Here's how the part is built. I have some questions about the finished solid (model axes, mm). A direction names the side the tool comes from. Round coordinates to 2 decimals unless told otherwise and drop trailing zeros. Write item = value, one per line. Start each with the question number.
Item 1: For faces 4 (the face through (33, -1.27, -17)), 5 (the face through (0.018, 27.397, 10.874)), 6 (the face through (-27.397, 0.018, 10.874)), 7 (the face through (-33, 1.27, -17)), which set-ups out of +Z, -Z, +X, -X, +Y, -Y let a thin tool reach every point of the face, with its end or its side?
Item 2: We'd pull the mould along Z, two halves only. Please class faces 1 (the face through (-6.21, -1.96, -88.74)), 2 (the face through (1.27, 33, -17)), 3 (the face through (-1.9, -8.7, -2.4)): pulls with the +Z half, pulls with the -Z half, needs draft (parallel to the pull), parting line crosses it, or undercut.
Item 3: I'm going to push flat-ended pins straight in: P1, Ø0.6, axis at x = 16.5, z = -102, coming from the -Y side; P2, Ø12.5, axis at x = 1.5, y = 4.5, coming from the +Z side; P3, Ø3, axis at x = 5.5, y = -32.5, coming from the +Z side. Where does each tip first touch, or does it pass through?
Item 4: Please list where these lines run through material, in increasing order: L1, parallel to X at y = 43.5, z = -3.5; L2, parallel to Z at x = 26, y = -9.
```python
from build123d import *

# Parameters (mm, degrees)
SKETCH2_R           = 8.763
CUT_EXTRUDE1_DEPTH  = 69.85
BOSS_EXTRUDE1_DEPTH = 1.27
CIRPATTERN1_COUNT   = 4
CHAMFER1_SIZE       = 2.54
SKETCH10_W          = 76.2
SKETCH10_H          = 76.2
BOSS_EXTRUDE4_DEPTH = 0.508


with BuildPart() as part:
    # Sketch1 → Revolve1 (revolve)
    with BuildSketch(Plane(origin=(0, 0, 0), x_dir=(1, 0, 0), z_dir=(0, 1, 0))):
        Polygon((0, 101.6), (-6.096, 101.6), (-6.096, 89.154), (-12.7, 82.55), (-12.7, 0), (0, 0), align=None)
    revolve(axis=Axis((0, 0, -101.6), (0, 0, 1)))

    # Sketch2 → Cut-Extrude1 (cut)
    with BuildSketch(Plane.XY):
        Circle(SKETCH2_R)
    extrude(amount=-CUT_EXTRUDE1_DEPTH, mode=Mode.SUBTRACT)

    # Sketch3 → Boss-Extrude1 (add, symmetric)
    with BuildSketch(Plane(origin=(0, 0, 0), x_dir=(1, 0, 0), z_dir=(0, 1, 0))):
        Polygon((-10.365704675, 0), (-12.7, 0), (-42.511621146, -22.056416192), (-58.358338046, -22.056416192), (-67.228379248, -13.18637499), (-67.228379248, -0.821064085), (-10.365704675, 79.063680635), align=None)
    boss_extrude1 = extrude(amount=BOSS_EXTRUDE1_DEPTH, both=True)

    # Cut-Sweep1: sweep along a path in Sketch4
    with BuildLine(Plane(origin=(-44.232547401, 0, -31.485122188), x_dir=(-0.579901297, 0, 0.814686741), z_dir=(-0.814686741, 0, -0.579901297))) as cut_sweep1_path:
        Line((39.654734318, 0), (-54.375714603, 0))
    # Sketch5 → Cut-Sweep1 (sweep, cut)
    with BuildSketch(Plane.ZY.offset(67.228379248)):
        with BuildLine():
            Line((8.176199828, -4.186863215), (8.176199828, -1.27))
            ThreePointArc((8.176199828, -1.27), (4.450761752, -0.912237677), (0.821064085, 0))
            ThreePointArc((0.821064085, 0), (4.450761752, 0.912237677), (8.176199828, 1.27))
            Line((8.176199828, 1.27), (8.176199828, 4.131781822))
            Line((8.176199828, 4.131781822), (-5.582166947, 4.131781822))
            Line((-5.582166947, 4.131781822), (-5.582166947, -4.186863215))
            Line((-5.582166947, -4.186863215), (8.176199828, -4.186863215))
        make_face()
    cut_sweep1 = sweep(path=cut_sweep1_path.line, mode=Mode.SUBTRACT)

    # CirPattern1: Boss-Extrude1, Cut-Sweep1 ×4 about axis
    cirpattern1_axis = Axis((0, 0, 38.786024747), (0, 0, -1))
    add([boss_extrude1.rotate(cirpattern1_axis, i * 360 / CIRPATTERN1_COUNT) for i in range(1, CIRPATTERN1_COUNT)])
    add([cut_sweep1.rotate(cirpattern1_axis, i * 360 / CIRPATTERN1_COUNT) for i in range(1, CIRPATTERN1_COUNT)], mode=Mode.SUBTRACT)

    # Sketch6 → Cut-Revolve1 (revolve, cut)
    with BuildSketch(Plane(origin=(0, 0, 0), x_dir=(1, 0, 0), z_dir=(0, 1, 0))):
        Polygon((-8.763, 69.85), (0, 85.027961227), (0, 69.85), align=None)
    revolve(axis=Axis((0, 0, -85.027961227), (0, 0, 1)), mode=Mode.SUBTRACT)

    # Chamfer1
    chamfer1_edges = [part.edges().sort_by_distance(p)[0] for p in [
        (-8.763, 0, 0),
    ]]
    chamfer(chamfer1_edges, length=CHAMFER1_SIZE)

    # Sketch10 → Boss-Extrude4 (add)
    with BuildSketch(Plane(origin=(0, 0, -101.6), x_dir=(-1, 0, 0), z_dir=(0, 0, -1))):
        Rectangle(SKETCH10_W, SKETCH10_H)
    extrude(amount=BOSS_EXTRUDE4_DEPTH)


solid = part.part
```
Filled in:
q1.face_4 = +Z, +X, -Y
q1.face_5 = +Z, +X, -X
q1.face_6 = +Z, +Y, -Y
q1.face_7 = +Z, -X, +Y
q2.face_1 = undercut
q2.face_2 = needs draft
q2.face_3 = pulls with the +Z half
q3.P1 = -38.1
q3.P2 = -0.31
q3.P3 = -101.6
q4.L1 = -1.27 to 1.27
q4.L2 = -102.11 to -101.6
